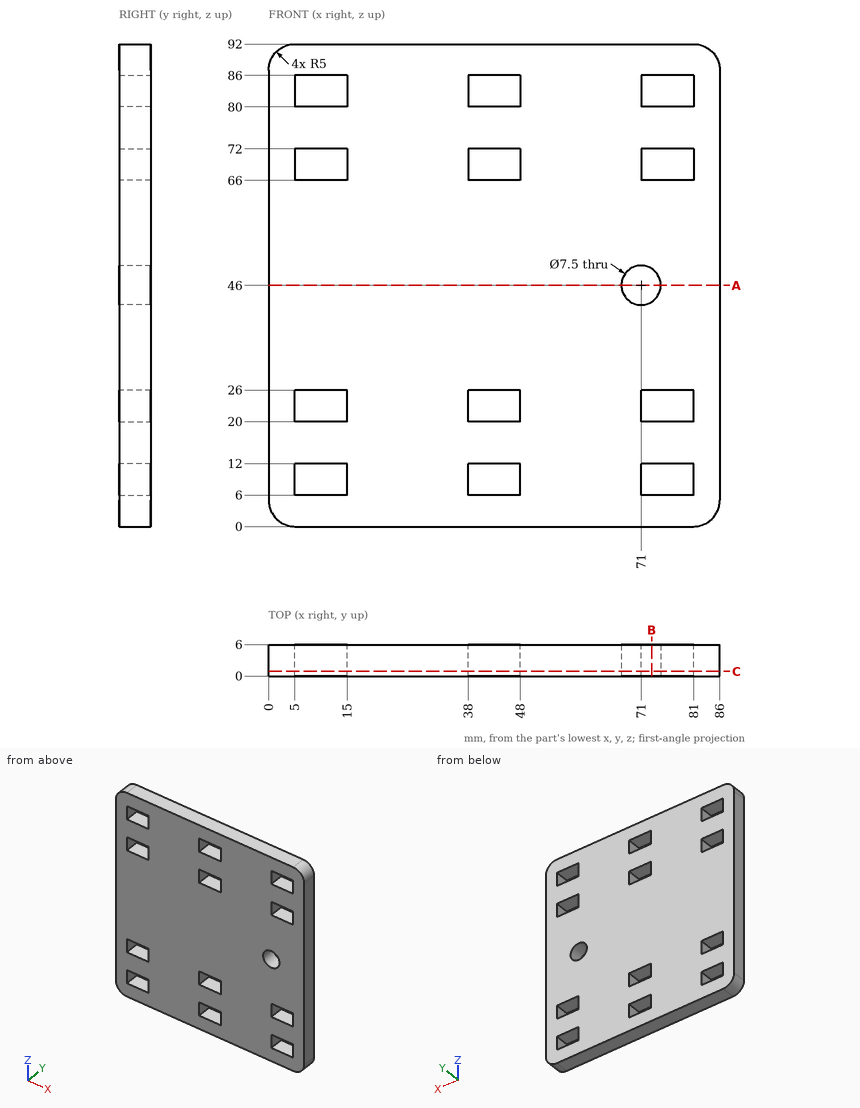
Could you check a few things on this drawing? It's one solid part, dimensions in mm from its lowest x, y, z. Give positions to 0.01 mm unless a question says otherwise; leave off trailing zeros. Order: outer loops, then holes, each group sorted by start corner. A loop starts at its lowest first (then second) coordinate and runs counter-clockwise, first axis right, second up.
1. Suppose I cut it at C-C (y = 0.9). State how many separate pieces and enclosed holes the cut face has, plus the area to 3 significant figures.
Answers below:
separate pieces: 1
enclosed holes: 13
area: 7,130 mm2
2. Suppose I cut it at A-A (z = 46). Write out the boundary of the cut face in (x, y), plus the area to 3 significant figures.
Answers below:
outline: (0, 0) - (67.25, 0) - (67.25, 6) - (0, 6) - close; (74.75, 0) - (86, 0) - (86, 6) - (74.75, 6) - close
area: 471 mm2
3. Suppose I cut it at B-B (x = 73). Write out the boundary of the cut face in (y, z).
Answers below:
outline: (0, 0) - (6, 0) - (6, 6) - (0, 6) - close; (0, 12) - (6, 12) - (6, 20) - (0, 20) - close; (0, 26) - (6, 26) - (6, 42.83) - (0, 42.83) - close; (0, 49.17) - (6, 49.17) - (6, 66) - (0, 66) - close; (0, 72) - (6, 72) - (6, 80) - (0, 80) - close; (0, 86) - (6, 86) - (6, 92) - (0, 92) - close
4. I need wall thicknesses on L1, parallel to X at y = 2.9, z = 82.5; L2, parallel to Z at x = 77.5, y = 3.35; L3, parallel to X at y = 4.5, z = 46. Which ranges of each line are inside material? Lowest first, please.
Answers below:
L1: x = 0 to 5, 15 to 38, 48 to 71, 81 to 86
L2: z = 0 to 6, 12 to 20, 26 to 66, 72 to 80, 86 to 92
L3: x = 0 to 67.25, 74.75 to 86
